```python
from build123d import *

# Parameters (mm, degrees)
BOSS_EXTRUDE1_START     = -60.5
BOSS_EXTRUDE1_OUTLINE_R = 2
BOSS_EXTRUDE1_DEPTH     = 121
SKETCH1_W               = 179.187175662
SKETCH1_H               = 206.234296517
SKETCH1_R               = 1.6025
SKETCH1_R_2             = 4
CUT_EXTRUDE1_DEPTH      = 80


# Read off the part's stored shape, not the designer's step: Boss-Extrude1
with BuildPart() as part:
    # Boss-Extrude1 outline → Boss-Extrude1 (new body)
    with BuildSketch(Plane(origin=(0, 0, 0), x_dir=(0, 0, -1), z_dir=(1, 0, 0)).offset(BOSS_EXTRUDE1_START)):
        with BuildLine():
            Line((6.0465, 72.85), (6.0465, 27.05))
            add(Edge.make_bspline(
                [(6.0465, 27.05), (6.0465, 21.716666667), (-15, 21.716666667), (-15, 11.05)],
                knots=[0, 0, 0, 0, 1, 1, 1, 1], degree=3))
            Line((-15, 11.05), (-15, -11.05))
            Line((-15, -11.05), (0, -11.05))
            Line((0, -11.05), (0, 11.05))
            add(Edge.make_bspline(
                [(0, 11.05), (0, 17.784890874), (36.209, 17.784890874)],
                knots=[0, 0, 0, 1, 1, 1], degree=2))
            Line((36.209, 17.784890874), (66.3715, 17.784890874))
            Line((66.3715, 17.784890874), (66.3715, 72.85))
            Line((66.3715, 72.85), (56.3715, 72.85))
            Line((56.3715, 72.85), (56.3715, 40.748146134))
            add(Edge.make_bspline(
                [(56.3715, 40.748146134), (56.3715, 25.284890874), (16.0465, 25.284890874), (16.0465, 40.748146134)],
                knots=[0, 0, 0, 0, 1, 1, 1, 1], degree=3))
            Line((16.0465, 40.748146134), (16.0465, 72.85))
            Line((16.0465, 72.85), (6.0465, 72.85))
        make_face()
        with Locations((11.0465, 35.516666667)):
            Circle(BOSS_EXTRUDE1_OUTLINE_R, mode=Mode.SUBTRACT)
        with Locations((11.0465, 69.383333333)):
            Circle(BOSS_EXTRUDE1_OUTLINE_R, mode=Mode.SUBTRACT)
        with Locations((61.3715, 35.516666667)):
            Circle(BOSS_EXTRUDE1_OUTLINE_R, mode=Mode.SUBTRACT)
        with Locations((61.3715, 69.383333333)):
            Circle(BOSS_EXTRUDE1_OUTLINE_R, mode=Mode.SUBTRACT)
    extrude(amount=BOSS_EXTRUDE1_DEPTH)

    # Sketch1 → Cut-Extrude1 (cut, symmetric)
    # profile 1 of 6: a face of its own
    with BuildSketch(Plane.XY):
        with Locations((-22.097828966, 29.224383364)):
            Rectangle(SKETCH1_W, SKETCH1_H)
        with BuildLine():
            add(Edge.make_bspline(
                [(0, -11.05), (54.05, 3.432653851), (54.05, 27.05)],
                knots=[0, 0, 0, 1, 1, 1], degree=2))
            Line((54.05, 27.05), (54.05, 72.85))
            Line((54.05, 72.85), (51.05, 72.85))
            Line((51.05, 72.85), (51.05, 27.05))
            add(Edge.make_bspline(
                [(0, 11.05), (51.05, 11.05), (51.05, 27.05)],
                knots=[0, 0, 0, 1, 1, 1], degree=2))
            ThreePointArc((0, 11.05), (-11.05, 0), (0, -11.05))
        make_face(mode=Mode.SUBTRACT)
    # profile 2 of 6: a face of its own
    with BuildSketch(Plane.XY):
        with Locations((8, 0)):
            Circle(SKETCH1_R)
    # profile 3 of 6: a face of its own
    with BuildSketch(Plane.XY):
        with Locations((0, 8)):
            Circle(SKETCH1_R)
    # profile 4 of 6: a face of its own
    with BuildSketch(Plane.XY):
        with Locations((-8, 0)):
            Circle(SKETCH1_R)
    # profile 5 of 6: a face of its own
    with BuildSketch(Plane.XY):
        with Locations((0, -8)):
            Circle(SKETCH1_R)
    # profile 6 of 6: a face of its own
    with BuildSketch(Plane.XY):
        Circle(SKETCH1_R_2)
    extrude(amount=CUT_EXTRUDE1_DEPTH, both=True, mode=Mode.SUBTRACT)


solid = part.part
```
Input: part model. Units: mm. Frame: model coordinates. A direction names the side the tool comes from. Give positions to 0.01 mm unless a question says otherwise; leave off trailing zeros. Order: outer loops, then holes, each group sorted by start corner. A loop starts at its lowest first (then second) coordinate and runs counter-clockwise, first axis right, second up. Notation, with made-up numbers: (84, -39.5) - (94, -39.5) arc R21 cw to (94, -19.5) - close; hole circle Ø1 at (-8.5, -2). An arc over 180 degrees is marked (long way). One line per item, written item: value.
1. Draft query along Z for faces 1 (the face through (53, 57, -56.372)), 2 (the face through (-0.21, 9.59, 7.4)), 3 (the face through (11, 3, 15)). Return one class per face: released by +Z, released by -Z, zero draft, split by the parting line, or undercut.
Determined:
face 1: undercut
face 2: zero draft
face 3: released by +Z
2. Cut plane A-A, the plane x = -8. Output: boundary loops of the cut face in (y, z).
Determined:
outline: (-7.62, 0) - (-1.6, 0) - (-1.6, 15) - (-7.62, 15) - close; (1.6, 0) - (7.62, 0) - (7.62, 15) - (1.6, 15) - close
3. Line query: probe 1 along X at (y, z) = (58.5, -56.5); probe 2 along X at (y, z) = (9, 10); probe 3 along Z at (x, y) = (37, 12). Output: solid intervals per line, ascending.
Determined:
probe 1: 51.05 to 54.05
probe 2: -6.41 to -1.25, 1.25 to 44.72
probe 3: -0.19 to 14.94
4. Cut plane B-B, the plane z = 1.5. Give the number of separate pieces and of enclosed holes in the cut face, and give its area (3 significant figures).
Determined:
separate pieces: 1
enclosed holes: 5
area: 868 mm2
5. Reachability of faces 4 (the face through (53, 50, -6.046)), 5 (the face through (52.5, 37.5, -10.8)), 6 (the face through (53, 57, -16.047)), 7 (the face through (48, 17.785, -51)) from +Z, -Z, +X, -X, +Y, -Y: full face, straight path, thin tool, end or side. Return the list, or none.
Determined:
face 4: +Z, +X, -X, +Y
face 5: +X, -X
face 6: +X, -X, +Y
face 7: -Z, +X, -X, -Y
6. Pin query (flat end, axial travel): pin 1 Ø4 at (x, y) = (0, -8) entering from -Z; pin 2 Ø4.5 at (y, z) = (69.38, -61.37) entering from -X; pin 3 Ø3.5 at (x, y) = (52, 55.5) entering from +Z. Return the tip coordinate at first contact, or that it passes through.
Determined:
pin 1: z = 0
pin 2: x = 51.05
pin 3: z = -6.05
